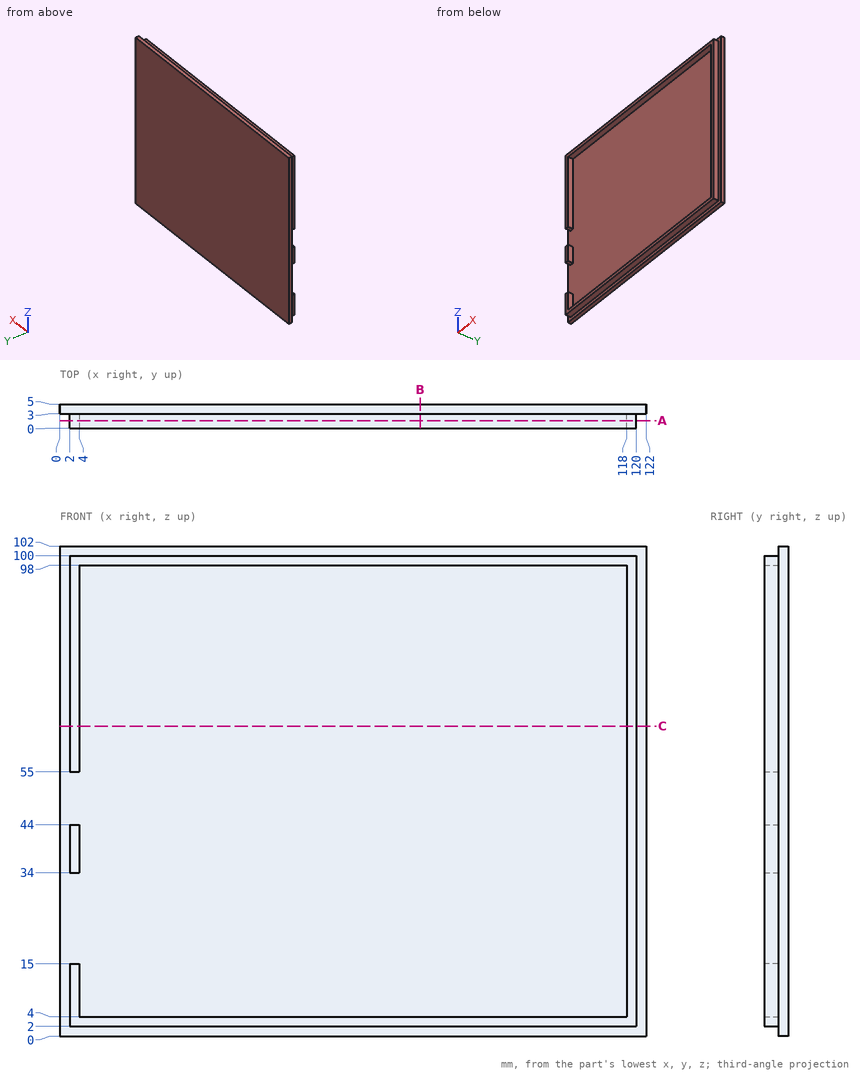
Can you work these out from the drawing? Everything is in mm from the part's minimum corner. Give positions to 0.01 mm unless a question says otherwise; leave off trailing zeros. Loops run counter-clockwise (first coordinate to the right, second up) from the corner with the lowest first, then second, coordinate; pieces in that order, holes last. Notation, with made-up numbers: (62, 39) -> (77, 39) arc R34 ccw to (77, 70) -> close; hole circle Ø9 at (75, 0.5). An arc over 180 degrees is marked (long way). Put each result on its own line as item: value.
(1) Imagine slicing it at B-B on x = 75. Write out the boundary of the cut face in (y, z), plus the area to 3 significant figures.
Computed:
outline: (0, 2) -> (3, 2) -> (3, 0) -> (5, 0) -> (5, 102) -> (3, 102) -> (3, 100) -> (0, 100) -> (0, 98) -> (3, 98) -> (3, 4) -> (0, 4) -> close
area: 216 mm^2
(2) Please list where these lines run through material, in increasing order: probe 1 along Z at (x, y) = (27.5, 2.7); probe 2 along X at (y, z) = (1.4, 9); probe 3 along Y at (x, z) = (112, 11). Write a range as [from, to].
Computed:
probe 1: [2, 4], [98, 100]
probe 2: [2, 4], [118, 120]
probe 3: [3, 5]
(3) Imagine slicing it at C-C on z = 64.5. Write out the boundary of the cut face in (x, y), plus the area to 3 significant figures.
Computed:
outline: (0, 3) -> (2, 3) -> (2, 0) -> (4, 0) -> (4, 3) -> (118, 3) -> (118, 0) -> (120, 0) -> (120, 3) -> (122, 3) -> (122, 5) -> (0, 5) -> close
area: 256 mm^2
(4) I'm going to push flat-ended pins straight in: pin 1 Ø5 at (x, z) = (104.5, 82) entering from -Y; pin 2 Ø1.5 at (y, z) = (1, 5.5) entering from -X; pin 3 Ø0.9 at (y, z) = (2, 39) entering from +X. Where does each tip first touch, or does it pass through?
Computed:
pin 1: y = 3
pin 2: x = 2
pin 3: x = 120
(5) Imagine slicing it at A-A on y = 1.55. Write out the boundary of the cut face in (x, z).
Computed:
outline: (2, 2) -> (120, 2) -> (120, 100) -> (2, 100) -> (2, 55) -> (4, 55) -> (4, 98) -> (118, 98) -> (118, 4) -> (4, 4) -> (4, 15) -> (2, 15) -> close; (2, 34) -> (4, 34) -> (4, 44) -> (2, 44) -> close
